Part model, mm, in its own coordinate system. A direction names the side the tool comes from. Coordinates: 2 decimals unless noted, no trailing zeros. Loops run counter-clockwise (first coordinate to the right, second up) from the corner with the lowest first, then second, coordinate; pieces in that order, holes last. Notation, with made-up numbers: (38, 44) -> (84, 44) arc R22 cw to (84, 63) -> close; hole circle Ø2 at (-14, 38.25). An arc over 180 degrees is marked (long way). Use one line per item in the form item = value. Start each with the question number.
(1) 3-axis set-ups, long thin cutter, end or side, ignore diameter. For faces 1 (the cylindrical face through (489.92, -2.17, -9.76)), 2 (the flat face through (-58, 0, 0)): which of +Z, -Z, +X, -X, +Y, -Y reach the whole face in a straight line?
(2) Pin check, flat tips, straight feed: P1, Ø7, axis at x = -19.5, y = -2, coming from the +Z side; P2, Ø1.5, axis at y = -15, z = -2.5, coming from the -X side; P3, Ø4.5, axis at x = -17.5, y = 1, coming from the -Z side. Stop position of each tip, or through.
(3) Drill centre lines: L1, parallel to X at y = 8, z = 13.5; L2, parallel to Z at x = 660, y = 4; L3, parallel to Y at x = 30, z = -2. Where is each one in solid material? Low to high. Write a range as [from, to].
(4) Band-saw the part on B-B on z = 20. Give the cut face in (x, y), then the cut area to 3 significant figures.
(5) Band-saw the part on C-C on y = 21.5. Give the cut face in (x, z), then the cut area to 3 significant figures.
(6) Band-saw the part on A-A on x = 741. Give the cut face in (y, z).
Autodesk Inventor part; units mm, degrees
ref_plane "K_XY" through (-14, 0, 0) normal (0, 0, 1) x (1, 0, 0)
ref_plane "K_YZ" through (-14, 0, 0) normal (1, 0, 0) x (0, 1, 0)
ref_plane "K_ZX" through (-14, 0, 0) normal (0, 1, 0) x (0, 0, 1)
sketch "Sketch_1" plane through (0, 0, 0) normal (0, 0, 1) x (1, 0, 0)
  line L0 (1002, 0) -> (-58, 0)
  line L1 (-58, 0) -> (-58, 8.08)
  line L2 (-58, 8.08) -> (-57.08, 9)
  line L3 (-57.08, 9) -> (-23, 9)
  line L4 (-23, 9) -> (-21.2679, 10)
  line L5 (-21.2679, 10) -> (987, 10)
  line L6 (987, 10) -> (987, 31.5)
  line L7 (987, 31.5) -> (1002, 31.5)
  line L8 (1002, 31.5) -> (1002, 0)
  line L9 (1002, 0) -> (-58, 0)
revolve "Revolution1" add sketch "Sketch_1" angle 360 about axis through (1002, 0, 0) along (1, 0, 0)
thread "Thread1"
sketch "Sketch_2" plane through (0, 0, 0) normal (0, 1, 0) x (-1, 0, 0)
  line L0 (23, -10) -> (23, -9)
  line L1 (23, -9) -> (14, -9)
  line L2 (14, -9) -> (13, -10)
  line L3 (13, -10) -> (23, -10)
extrude "Extrusion1" cut sketch "Sketch_2" along normal mid plane 20
sketch "Sketch_3" plane through (0, 0, 0) normal (0, 1, 0) x (-1, 0, 0)
  line L0 (23, 10) -> (13, 10)
  line L1 (13, 10) -> (14, 9)
  line L2 (14, 9) -> (23, 9)
  line L3 (23, 9) -> (23, 10)
extrude "Extrusion2" cut sketch "Sketch_3" along normal mid plane 20
ref_plane "K_XY" through (-14, 0, 0) normal (0, 0, 1) x (1, 0, 0)
ref_plane "K_YZ" through (-14, 0, 0) normal (1, 0, 0) x (0, 1, 0)
ref_plane "K_ZX" through (-14, 0, 0) normal (0, 1, 0) x (0, 0, 1)
ref_plane "rod_XY" through (0, 0, 0) normal (1, 0, 0) x (0, 0, -1)
ref_plane "rod_YZ" through (0, 0, 0) normal (0, 0, -1) x (0, 1, 0)
ref_plane "rod_ZX" through (0, 0, 0) normal (0, 1, 0) x (1, 0, 0)
ref_plane "rod_nut_XY" through (-42, 0, 0) normal (-1, 0, 0) x (0, 0, -1)
ref_plane "rod_nut_YZ" through (-42, 0, 0) normal (0, 0, -1) x (0, -1, 0)
ref_plane "rod_nut_ZX" through (-42, 0, 0) normal (0, -1, 0) x (-1, 0, 0)
properties part number "CE263-800_ROD"
A:
q1.face_1 = -X
q1.face_2 = +Z, -Z, -X, +Y, -Y
q2.P1 = 9
q2.P2 = 987
q2.P3 = -9
q3.L1 = [987, 1002]
q3.L2 = [-9.17, 9.17]
q3.L3 = [-9.8, 9.8]
q4.outline = (987, -24.34) -> (1002, -24.34) -> (1002, 24.34) -> (987, 24.34) -> close
q4.area = 730 mm²
q5.outline = (987, -23.02) -> (1002, -23.02) -> (1002, 23.02) -> (987, 23.02) -> close
q5.area = 691 mm²
q6.outline = circle Ø20 at (0, 0)
